Read the model definition and answer for the solid it produces. Units are mm, in the model's axes. A direction names the side the tool comes from. Give positions to 0.01 mm unless a question says otherwise; leave off trailing zeros. Loops run counter-clockwise (first coordinate to the right, second up) from the corner with the lowest first, then second, coordinate; pieces in that order, holes last.
(1) Find section D-D, the plane x = 267. Write down the section's boundary in (y, z), then the cut area to 3 significant figures.
(2) Determine the mould class of faces 4 (the face through (44, -25, 9)), 5 (the face through (344, 22, 0)), 6 (the face through (134.726, -24.787, -3.255)) for opening direction Z: pulls with the +Z half, pulls with the -Z half, needs draft (parallel to the pull), parting line crosses it, or undercut.
(3) Straight lines are drawn through the part: probe 1 along Y at (x, z) = (159, 1); probe 2 along X at (y, z) = (24, -3); probe 3 along X at (y, z) = (-6.5, -24). For each, find the intervals that lie inside material, in ascending order.
(4) Find section B-B, the plane x = 168. Write down the section's boundary in (y, z), then the cut area to 3 significant figures.
(5) Each of these flat-tipped pins is pushed along its axis until it touches: P1, Ø3.5, axis at x = 77, y = 20.5, coming from the +Z side; P2, Ø10, axis at x = 235.5, z = 22, coming from the -Y side; P3, Ø1.4, axis at x = 311, y = 22.5, coming from the -Z side. Where does it stop, or does it pass through?
(6) Find section C-C, the plane x = 25. Write down the section's boundary in (y, z), then the cut area to 3 significant figures.
(7) Which of the six approach directions +Z, -Z, +X, -X, +Y, -Y give full straight-line access (tool end or side, diameter ignored) to faces 1 (the face through (4, 20.3, -11)), 2 (the face through (46, 22, 0)), 3 (the face through (22, -25, -7))?
```python
from build123d import *

# Parameters (mm, degrees)
CUT_EXTRUDE1_DEPTH = 6
CUT_EXTRUDE2_DEPTH = 6
FILLET1_R          = 1
CUT_EXTRUDE3_DEPTH = 6


with BuildPart() as part:
    # Sketch1 → Revolve1 (revolve)
    with BuildSketch(Plane.XY, mode=Mode.PRIVATE) as revolve1_sk:
        Polygon((0, 0), (349, 0), (349, 23), (347, 25), (229, 25), (229, 22.9), (227, 22.9), (227, 25), (44, 25), (44, 30), (22, 30), (22, 25), (6, 25), (6, 22.9), (4, 22.9), (4, 25), (2, 25), (0, 23), align=None)
    revolve(revolve1_sk.sketch.rotate(Axis((0, 0, 0), (1, 0, 0)), 90), axis=Axis((0, 0, 0), (1, 0, 0)))

    # Sketch2 → Cut-Extrude1 (cut)
    with BuildSketch(Plane(origin=(0, 25, 0), x_dir=(1, 0, 0), z_dir=(0, 1, 0))):
        with BuildLine():
            Line((54, 8), (94, 8))
            ThreePointArc((94, 8), (102, 0), (94, -8))
            Line((94, -8), (54, -8))
            ThreePointArc((54, -8), (46, 0), (54, 8))
        make_face()
    extrude(amount=-CUT_EXTRUDE1_DEPTH, mode=Mode.SUBTRACT)

    # Sketch3 → Cut-Extrude2 (cut)
    with BuildSketch(Plane(origin=(0, 25, 0), x_dir=(1, 0, 0), z_dir=(0, 1, 0))):
        with BuildLine():
            Line((124.5, 8), (178.5, 8))
            ThreePointArc((178.5, 8), (186.5, 0), (178.5, -8))
            Line((178.5, -8), (124.5, -8))
            ThreePointArc((124.5, -8), (116.5, 0), (124.5, 8))
        make_face()
    extrude(amount=-CUT_EXTRUDE2_DEPTH, mode=Mode.SUBTRACT)

    # Fillet1
    fillet1_edges = [part.edges().sort_by_distance(p)[0] for p in [
        (44, 0, -25),
    ]]
    fillet(fillet1_edges, radius=FILLET1_R)

    # Sketch4 → Cut-Extrude3 (cut)
    with BuildSketch(Plane(origin=(0, 25, 0), x_dir=(1, 0, 0), z_dir=(0, 1, 0))):
        with BuildLine():
            Line((296, 8), (336, 8))
            ThreePointArc((336, 8), (344, 0), (336, -8))
            Line((336, -8), (296, -8))
            ThreePointArc((296, -8), (288, 0), (296, 8))
        make_face()
    extrude(amount=-CUT_EXTRUDE3_DEPTH, mode=Mode.SUBTRACT)


solid = part.part
```
Entries:
1. outline: circle Ø50 at (0, 0)
1. area: 1,960 mm2
2. face 4: needs draft
2. face 5: undercut
2. face 6: parting line crosses it
3. probe 1: y = -24.98 to 19
3. probe 2: x = 1.19 to 4, 6 to 46.58, 101.42 to 117.08, 185.92 to 227, 229 to 288.58, 343.42 to 347.81
3. probe 3: x = 1.86 to 4, 6 to 227, 229 to 347.14
4. outline: (19, -8) - (19, 8) - (23.69, 8) arc R25 ccw (long way) to (23.69, -8) - close
4. area: 1,870 mm2
5. P1: stops at z = 16.54
5. P2: stops at y = -18.33
5. P3: stops at z = -12.24
6. outline: circle Ø60 at (0, 0)
6. area: 2,830 mm2
7. face 1: none
7. face 2: +Y
7. face 3: -X
